Job drawing, mm, ordinate dimensions from the low corner. One solid piece. Round coordinates to 2 decimals unless told otherwise and drop trailing zeros. Loops run counter-clockwise (first coordinate to the right, second up) from the corner with the lowest first, then second, coordinate; pieces in that order, holes last. Notation, with made-up numbers: M 53.5,-27 L 61.5,-27 A36 ccw 61.5,11 Z; hole C 5,82.25 d7. An arc over 180 degrees is marked long. Use a Markdown table: item, result. Add a question column.
(1) Two-plate mould, pull along X, no slides. Class the marked faces 1, 2, 3 and 4: released by +X, released by -X, zero draft, split by the parting line, or undercut.
(2) Flat gauge pin, fed straight in: P1, Ø0.9, axis at y = 2.5, z = 2, coming from the -X side. Where does the tip first touch, or does it go through?
(3) Band-saw the part on A-A, the plane z = 15.5. Write the cut outline in (x, y), and give its area (3 significant figures).
(4) Band-saw the part on C-C, the plane y = 4.2. Give the number of separate pieces and of enclosed holes in the cut face, and give its area (3 significant figures).
(5) Band-saw the part on B-B, the plane x = 17.5. Write the cut outline in (y, z), and give its area (3 significant figures).
(6) Wall check: L1, parallel to X at y = 5.3, z = 5.5; L2, parallel to X at y = 1, z = 21.5; L3, parallel to Z at x = 11, y = 3.85. Give the ranges that are in metal, low to high.
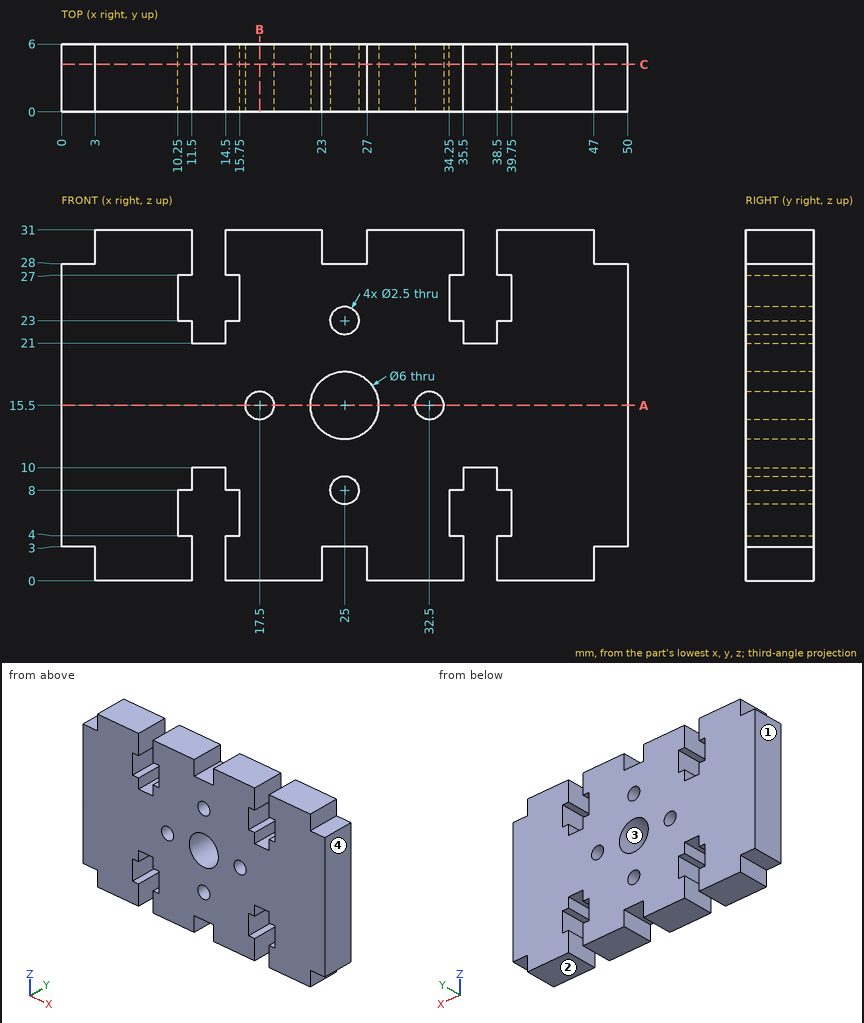
Return value:
| question | item | result |
|---|---|---|
| 1 | face 1 | released by -X |
| 1 | face 2 | zero draft |
| 1 | face 3 | undercut |
| 1 | face 4 | released by +X |
| 2 | P1 | x = 3 |
| 3 | outline | M 0,0 L 16.25,0 L 16.25,6 L 0,6 Z; M 18.75,0 L 22,0 L 22,6 L 18.75,6 Z; M 28,0 L 31.25,0 L 31.25,6 L 28,6 Z; M 33.75,0 L 50,0 L 50,6 L 33.75,6 Z |
| 3 | area | 234 mm^2 |
| 4 | separate pieces | 1 |
| 4 | enclosed holes | 5 |
| 4 | area | 1,280 mm^2 |
| 5 | outline | M 0,0 L 6,0 L 6,14.25 L 0,14.25 Z; M 0,16.75 L 6,16.75 L 6,31 L 0,31 Z |
| 5 | area | 171 mm^2 |
| 6 | L1 | 0 to 10.25, 15.75 to 34.25, 39.75 to 50 |
| 6 | L2 | 0 to 11.5, 14.5 to 35.5, 38.5 to 50 |
| 6 | L3 | 0 to 4, 8 to 23, 27 to 31 |
